```python
from build123d import *

# Parameters (mm, degrees)
EXTRUDE1_DEPTH     = 12.7
SKETCH2_R          = 3.96875
CUT_EXTRUDE1_DEPTH = 162.863978698
SKETCH3_W          = 12.7
SKETCH3_H          = 12.7
EXTRUDE2_DEPTH     = 162.863978698
SKETCH4_W          = 105.983052191
SKETCH4_H          = 75.202262717
EXTRUDE3_DEPTH     = 162.863978698


with BuildPart() as part:
    # Sketch1 → Extrude1 (new body)
    with BuildSketch(Plane.XY):
        with BuildLine():
            Line((-76.2, 12.7), (-53.975, 12.7))
            Line((-53.975, 12.7), (-53.975, 0))
            Line((-53.975, 0), (-34.925, 0))
            Line((-34.925, 0), (-34.925, 12.7))
            Line((-34.925, 12.7), (34.925, 12.7))
            Line((34.925, 12.7), (34.925, 0))
            Line((34.925, 0), (53.975, 0))
            Line((53.975, 0), (53.975, 12.7))
            Line((53.975, 12.7), (76.2, 12.7))
            Line((76.2, 12.7), (76.2, 142.24))
            Line((76.2, 142.24), (63.5, 142.24))
            ThreePointArc((63.5, 142.24), (0, 78.74), (-63.5, 142.24))
            Line((-63.5, 142.24), (-76.2, 142.24))
            Line((-76.2, 142.24), (-76.2, 12.7))
        make_face()
    extrude(amount=EXTRUDE1_DEPTH)

    # Sketch2 → Cut-Extrude1 (cut, through all)
    with BuildSketch(Plane.XY.offset(12.7)):
        with Locations((44.45, 66.04)):
            Circle(SKETCH2_R)
    extrude(amount=-CUT_EXTRUDE1_DEPTH, mode=Mode.SUBTRACT)

    # Sketch3 → Extrude2 (cut, through all)
    with BuildSketch(Plane.XY.offset(12.7)):
        with Locations((-69.85, 19.05)):
            Rectangle(SKETCH3_W, SKETCH3_H)
    extrude(amount=-EXTRUDE2_DEPTH, mode=Mode.SUBTRACT)

    # Sketch4 → Extrude3 (cut, through all)
    with BuildSketch(Plane.XY.offset(12.7)):
        with Locations((52.991526096, 116.341131359)):
            Rectangle(SKETCH4_W, SKETCH4_H)
    extrude(amount=-EXTRUDE3_DEPTH, mode=Mode.SUBTRACT)


solid = part.part
```
Verification items for the finished model (mm, model axes). A direction names the side the tool comes from. Round coordinates to 2 decimals unless told otherwise and drop trailing zeros. Write each loop counter-clockwise with the first axis right and the second up, starting at its lowest first coordinate (ties: lowest second). Pieces come first, ordered by that corner, then holes. Notation, with made-up numbers: (12, -26.5) - (36, -26.5) arc R22 ccw to (36, 1.5) - close; hole circle Ø9 at (11.5, -39). An arc over 180 degrees is marked (long way). Answer as a JSON object with one key per item and string values. Group by question number.
Q1. Section check B-B, the plane x = 44.45. Enter the section's corners in (y, z), plus the area to 3 significant figures.
Q2. Tool access check on faces 1 (the flat face through (65, 12.7, 6)), 2 (the flat face through (-34.925, 6, 6)), 3 (the flat face through (38, 78.74, 6)), 4 (the flat face through (-59, 12.7, 6)). Record the directions out of +Z, -Z, +X, -X, +Y, -Y that give a thin tool (end or side, any length) a straight path to the whole face; none if there is none.
Q3. Mould release check, pull along X, two halves, no side actions. Record for faces 5 (the flat face through (-45, 0, 6)), 6 (the flat face through (-53.975, 6, 6)), 7 (the flat face through (0, 12.7, 6)), 8 (the flat face through (76.2, 45, 6)): released by +X, released by -X, zero draft, split by the parting line, or undercut.
Q4. Section check A-A, the plane y = 11. Enter the section's corners in (x, z) (3 decimals), plus the area to 3 significant figures.
Q5. Thickness scan on line 1 (Y direction, x = 44.45, z = 3); line 2 (Y direction, x = 55, z = 11); line 3 (X direction, y = 64.5, z = 6). Record the ranges inside material, lowest first.
Q6. Section check D-D, the plane y = 132.5. Enter the section's corners in (x, z), plus the area to 3 significant figures.
Q7. Go/stop test with flat-tipped pins: pin 1 Ø6 at (x, y) = (-19, 87.5) entering from +Z; pin 2 Ø4 at (x, z) = (39, 5.5) entering from +Y; pin 3 Ø7.5 at (x, z) = (-60, 9) entering from -Y; pin 4 Ø4 at (x, z) = (-70, 7.5) entering from -Y. Record where each tip stops, or that it passes through.
Found:
{
 "1": {"outline": "(0, 0) - (62.07, 0) - (62.07, 12.7) - (0, 12.7) - close; (70.01, 0) - (78.74, 0) - (78.74, 12.7) - (70.01, 12.7) - close", "area": "899 mm^2"},
 "2": {"face 1": "+Z, -Z, +X, -Y", "face 2": "+Z, -Z, -Y", "face 3": "+Z, -Z, +X, +Y", "face 4": "+Z, -Z, -X, -Y"},
 "3": {"face 5": "zero draft", "face 6": "released by -X", "face 7": "undercut", "face 8": "released by +X"},
 "4": {"outline": "(-53.975, 0) - (-34.925, 0) - (-34.925, 12.7) - (-53.975, 12.7) - close; (34.925, 0) - (53.975, 0) - (53.975, 12.7) - (34.925, 12.7) - close", "area": "484 mm^2"},
 "5": {"line 1": "y = 0 to 62.07, 70.01 to 78.74", "line 2": "y = 12.7 to 78.74", "line 3": "x = -76.2 to 40.79, 48.11 to 76.2"},
 "6": {"outline": "(-76.2, 0) - (-62.75, 0) - (-62.75, 12.7) - (-76.2, 12.7) - close", "area": "171 mm^2"},
 "7": {"pin 1": "passes through", "pin 2": "stops at y = 78.74", "pin 3": "stops at y = 12.7", "pin 4": "stops at y = 25.4"}
}
